```python
from build123d import *

# Parameters (mm, degrees)
SKETCH1_W           = 40
SKETCH1_H           = 20
BOSS_EXTRUDE1_DEPTH = 40
CUT_EXTRUDE18_DEPTH = 20
CUT_EXTRUDE20_DEPTH = 59
CUT_EXTRUDE21_DEPTH = 59


with BuildPart() as part:
    # Sketch1 → Boss-Extrude1 (new body)
    with BuildSketch(Plane.XY):
        with BuildLine():
            Line((0, 20), (40, 20))
            ThreePointArc((40, 20), (20, 40), (0, 20))
        make_face()
        with Locations((20, 10)):
            Rectangle(SKETCH1_W, SKETCH1_H)
    extrude(amount=BOSS_EXTRUDE1_DEPTH)

    # Sketch4 → Cut-Extrude18 (cut)
    with BuildSketch(Plane.XY.offset(40)):
        with BuildLine():
            Line((20, 30), (20, 20))
            Line((20, 20), (10, 20))
            ThreePointArc((10, 20), (12.928932188, 27.071067812), (20, 30))
        make_face()
    extrude(amount=-CUT_EXTRUDE18_DEPTH, mode=Mode.SUBTRACT)

    # Sketch11 → Cut-Extrude20 (cut)
    with BuildSketch(Plane(origin=(0, 0, 0), x_dir=(1, 0, 0), z_dir=(0, 1, 0))):
        Polygon((20, -40), (0, 0), (0, -40), align=None)
        Polygon((40, 0), (20, -40), (40, -40), align=None)
    extrude(amount=CUT_EXTRUDE20_DEPTH, mode=Mode.SUBTRACT)

    # Sketch12 → Cut-Extrude21 (cut)
    with BuildSketch(Plane(origin=(0, 0, 0), x_dir=(0, 0, -1), z_dir=(1, 0, 0))):
        Polygon((-40, 20), (0, 40), (-40, 40), align=None)
    extrude(amount=CUT_EXTRUDE21_DEPTH, mode=Mode.SUBTRACT)


solid = part.part
```
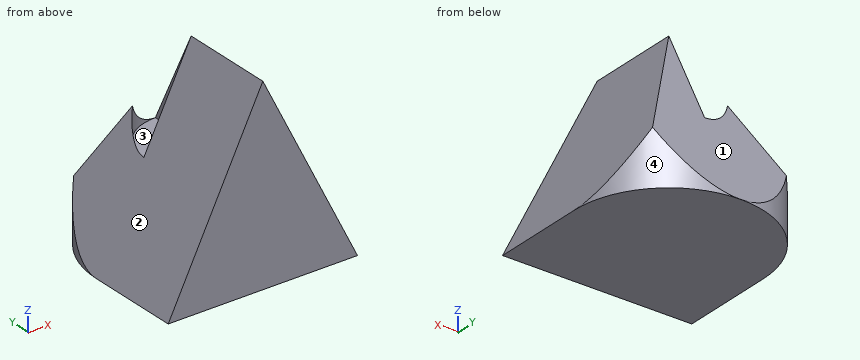
Can you work these out from the model? Positions are in its coordinate system, mm. Face numbers are marked on the shaded views. Give positions to 0.01 mm unless a question says otherwise; leave off trailing zeros. Loops run counter-clockwise (first coordinate to the right, second up) from the corner with the lowest first, then second, coordinate; pieces in that order, holes last. Notation, with made-up numbers: M -36,5 L 20,5 A23 cw 20,18 Z; hole C 48.5,67 d7. An arc over 180 degrees is marked long. One line per item, written item: value.
(1) Suppose I cut it at C-C on y = 21. List the corners of the cut face in (x, z) for me.
Returned:
outline: M 0.03,0 L 39.97,0 L 39.97,0.05 L 21,38 L 20,38 L 20,20 L 10.05,20 L 10.05,20.1 L 0.03,0.05 Z
(2) Suppose I cut it at D-D on x = 30. List the corners of the cut face in (y, z) for me.
Returned:
outline: M 0,0 L 37.32,0 L 37.32,5.36 L 30,20 L 0,20 Z
(3) Will these pins go through, and if not, where does the flat tip stop? pin 1 (3 mm diameter, centred on y = 26, z = 30, fed in from -X); pin 2 (8 mm diameter, centred on y = 13, z = 33, fed in from +X); pin 3 (1 mm diameter, centred on x = 18, z = 7, fed in from +Y).
Returned:
pin 1: x = 20
pin 2: x = 25.5
pin 3: y = 36.75
(4) Suppose I cut it at B-B on z = 37. List the corners of the cut face in (x, y) for me.
Returned:
outline: M 18.5,0 L 21.5,0 L 21.5,21.5 L 20,21.5 L 20,20 L 18.5,20 Z
(5) Suppose I cut it at A-A on z = 21. List the corners of the cut face in (x, y) for me.
Returned:
outline: M 10.5,0 L 29.5,0 L 29.5,29.5 L 20,29.5 L 20,20 L 10.5,20 Z; M 10.5,23.12 A10 cw 16.88,29.5 L 10.5,29.5 Z
(6) We'd pull the mould along X, two halves only. Please class the marked faces 1, 2, 3 and 4: released by +X, released by -X, zero draft, split by the parting line, or undercut.
Returned:
face 1: zero draft
face 2: released by -X
face 3: undercut
face 4: released by +X
(7) I need wall thicknesses on line 1 (Z direction, x = 5, y = 27); line 2 (Z direction, x = 2, y = 28); line 3 (Y direction, x = 17.5, z = 12.5). Which ranges of each line are inside material? Lowest first, please.
Returned:
line 1: 0 to 10
line 2: 0 to 4
line 3: 0 to 33.75
